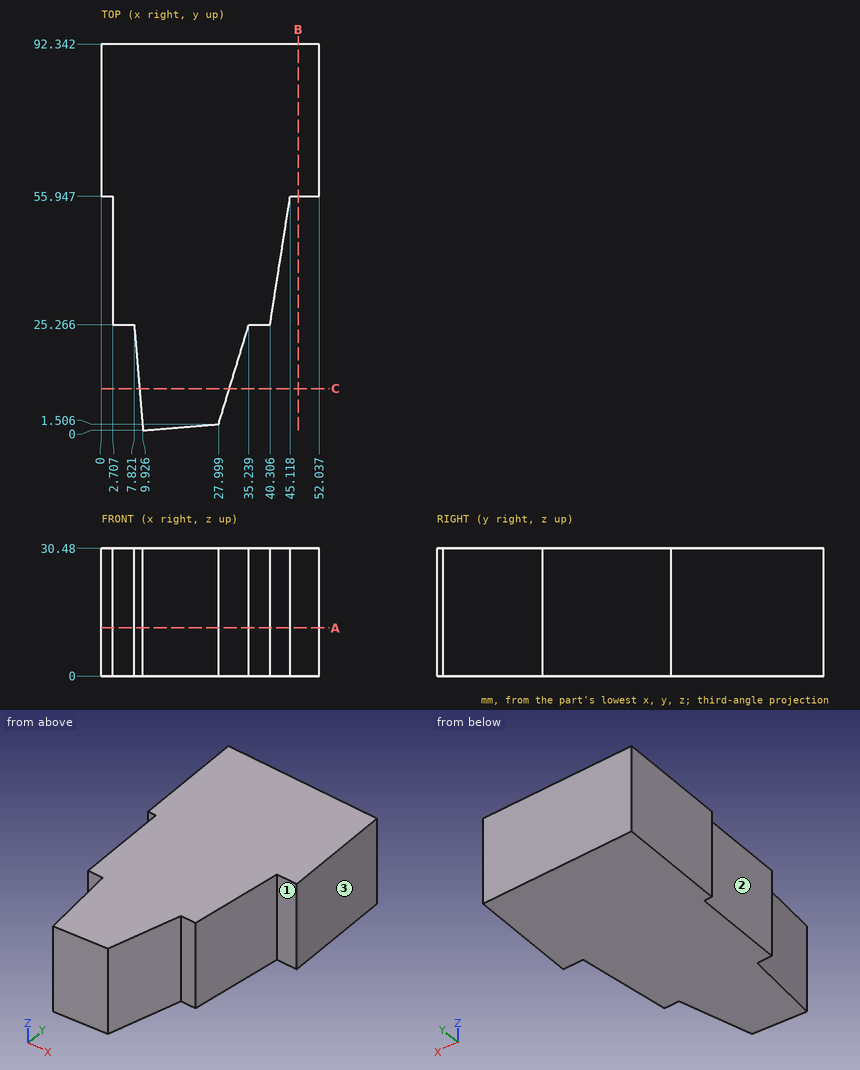
Check sheet for the drawn part. Datum: minimum x, y, z corner. Units: mm. A direction names the side the tool comes from. Round coordinates to 2 decimals unless told otherwise and drop trailing zeros. Order: outer loops, then holes, each group sorted by start corner. A loop starts at its lowest first (then second) coordinate and runs counter-clockwise, first axis right, second up. Notation, with made-up numbers: M 14,46.5 L 62,46.5 A14 cw 62,64.5 Z; hole C 84,78.25 d5. An arc over 180 degrees is marked long. Answer in a Markdown table with one row per item.
(1) Material ranges on line 1 along Y through (x, z) = (47, 5.5); line 2 along Y through (x, z) = (37.5, 12); line 3 along X through (y, z) = (21.5, 24.5) (1 decimal), recorded low to high. Write a range as from..to.
Findings:
| item | result |
|---|---|
| line 1 | y = 55.95..92.34 |
| line 2 | y = 25.27..92.34 |
| line 3 | x = 8.1..34.1 |
(2) Section check C-C on y = 10. Record the boundary of the cut face in (x, z).
Findings:
| item | result |
|---|---|
| outline | M 9.09,0 L 30.59,0 L 30.59,30.48 L 9.09,30.48 Z |
(3) Gauge pin test, flat ends, axial feed: pin 1 (7.5 mm diameter, centred on x = 50, z = 10, fed in from -Y); pin 2 (1 mm diameter, centred on y = 41, z = 6, fed in from +X); pin 3 (5 mm diameter, centred on y = 26.5, z = 26.5, fed in from +X). Record the tip position at first contact, or that the pin passes through.
Findings:
| item | result |
|---|---|
| pin 1 | stops at y = 55.95 |
| pin 2 | stops at x = 42.85 |
| pin 3 | stops at x = 40.89 |
(4) Section check A-A on z = 11.5. Record the boundary of the cut face in (x, y) (1 decimal).
Findings:
| item | result |
|---|---|
| outline | M 0,55.9 L 2.7,55.9 L 2.7,25.3 L 7.8,25.3 L 9.9,0 L 28,1.5 L 35.2,25.3 L 40.3,25.3 L 45.1,55.9 L 52,55.9 L 52,92.3 L 0,92.3 Z |
(5) Set-up check for the marked faces 1, 2 and 3: record each of +Z, -Z, +X, -X, +Y, -Y from which the full face is reachable in a straight line by a thin tool's end or side.
Findings:
| item | result |
|---|---|
| face 1 | +Z, -Z, +X, -Y |
| face 2 | +Z, -Z, -X, -Y |
| face 3 | +Z, -Z, +X, +Y, -Y |
(6) Section check B-B on x = 47. Record the boundary of the cut face in (y, z).
Findings:
| item | result |
|---|---|
| outline | M 55.95,0 L 92.34,0 L 92.34,30.48 L 55.95,30.48 Z |
